from build123d import *

# Parameters (mm, degrees)
F0_R     = 11.2
F2_DEPTH = 7
F3_R     = 1.5
F4_R     = 1.5


with BuildPart() as f2:
    # F0 (on Top) → F2 (new body)
    with BuildSketch(Plane.XY):
        with BuildLine():
            Line((13.200049, -27.049193), (13.133245, -1.325845))
            Line((13.133245, -1.325845), (13.126182, 1.394041))
            Line((13.126182, 1.394041), (13.064269, 25.233856))
            ThreePointArc((13.064269, 25.233856), (-0.000644, 40.321941), (-13.064085, 25.232581))
            Line((-13.064085, 25.232581), (-13.125989, 1.395851))
            Line((-13.125989, 1.395851), (-13.133062, -1.327656))
            Line((-13.133062, -1.327656), (-13.199862, -27.049193))
            ThreePointArc((-13.199862, -27.049193), (9.4e-05, -40.283473), (13.200049, -27.049193))
        make_face()
        Circle(F0_R, mode=Mode.SUBTRACT)
        with Locations((9.4e-05, -27.083473)):
            Circle(F0_R, mode=Mode.SUBTRACT)
        with Locations((0, 27.121941)):
            Circle(F0_R, mode=Mode.SUBTRACT)
    extrude(amount=F2_DEPTH)

    # F3
    f3_edges = [f2.edges().sort_by_distance(p)[0] for p in [
        (13.132159, -0.907668, 7),
        (9.4e-05, -40.283473, 7),
        (-13.131973, -0.908306, 7),
        (-0.000644, 40.321941, 7),
    ]]
    fillet(f3_edges, radius=F3_R)

    # F4
    f4_edges = [f2.edges().sort_by_distance(p)[0] for p in [
        (-0.000644, 40.321941, 0),
        (13.132159, -0.907668, 0),
        (-13.131973, -0.908306, 0),
        (9.4e-05, -40.283473, 0),
    ]]
    fillet(f4_edges, radius=F4_R)


solid = f2.part
Build history of the part. All positions in model axes, mm. Coordinates: 2 decimals unless noted, no trailing zeros. Order: outer loops, then holes, each group sorted by start corner. A loop starts at its lowest first (then second) coordinate and runs counter-clockwise, first axis right, second up. Notation, with made-up numbers: (47.25, 41) -> (89.25, 41) arc R21 ccw to (89.25, 75) -> close; hole circle Ø5 at (17.25, -10.5). An arc over 180 degrees is marked (long way). One line per item, written item: value.
(1) Probe line 1 (Y direction, x = 0, z = 3.25); line 2 (Y direction, x = -2.75, z = 1); line 3 (X direction, y = -21.5, z = 1.5). List the from-to ranges inside material, lowest first. Write a range as [from, to].
Checked values:
line 1: [-40.28, -38.28], [-15.88, -11.2], [11.2, 15.92], [38.32, 40.32]
line 2: [-39.91, -37.94], [-16.23, -10.86], [10.86, 16.26], [37.98, 39.94]
line 3: [-13.19, -9.71], [9.71, 13.19]
(2) Slice it at A-A, the plane x = 0. Count the separate pieces of the cut face and the enclosed holes in it, plus the area to 3 significant figures.
Checked values:
separate pieces: 4
enclosed holes: 0
area: 91.9 mm2
(3) Drop flat-ended pins along their axis: pin 1 Ø1.5 at (x, z) = (-1.5, 1) entering from +Y; pin 2 Ø2 at (y, z) = (-21.5, 3.5) entering from -X; pin 3 Ø4 at (x, z) = (-8.5, 4.5) entering from -Y. Give the stop position or say it passes through.
Checked values:
pin 1: y = 40.29
pin 2: x = -13.19
pin 3: y = -38.57
(4) Slice it at B-B, the plane z = 3.5. List the corners of the cut face in (x, y), plus the area to 3 significant figures.
Checked values:
outline: (-13.2, -27.05) arc R13.2 ccw to (13.2, -27.05) -> (13.13, -1.33) -> (13.13, 1.39) -> (13.06, 25.23) arc R13.2 ccw (long way) to (-13.06, 25.23) -> close; hole circle Ø22.4 at (0, -27.08); hole circle Ø22.4 at (0, 0); hole circle Ø22.4 at (0, 27.12)
area: 789 mm2
(5) Mould opens along X. For faces 1 (the cylindrical face through (-0.29, -40.28, 3.47)), 2 (the flat face through (-1.8, -11.3, 0)), 3 (the cylindrical face through (-1.458, 38.227, 3.451)) say: pulls with the +X half, pulls with the -X half, needs draft (parallel to the pull), parting line crosses it, or undercut.
Checked values:
face 1: parting line crosses it
face 2: needs draft
face 3: undercut
